For this review, take the finished solid that the model builds, in its own axes (mm). A direction names the side the tool comes from. Coordinates: 2 decimals unless noted, no trailing zeros. Loops run counter-clockwise (first coordinate to the right, second up) from the corner with the lowest first, then second, coordinate; pieces in that order, holes last. Notation, with made-up numbers: M -21.75,-28.5 L 17.25,-28.5 A21 cw 17.25,-12.5 Z; hole C -26,-34.75 d4. An arc over 180 degrees is marked long. Answer as a JSON object with one key per item and string values. Group by question number.
Item 1: Tool access review of faces 4 (the face through (6.35, 121, 10)), 5 (the face through (3, 86.995, 13)), 6 (the face through (24.99, 5.63, -55.48)): name each direction out of +Z, -Z, +X, -X, +Y, -Y from which nothing blocks a thin tool from reaching the whole face with its end or side.
Item 2: Wall thickness on L1, parallel to X at y = 66.5, z = -83; L2, parallel to Z at x = 23, y = 29.5: over which ranges is each line inside the solid? List them lowest first. Write a range as from..to.
Item 3: Add section D-D (y = 56.5). State the section outline as (x, z) points, then the cut area to 3 significant figures.
Item 4: Add section B-B (z = 4.5). State the section outline as (x, y) points (3 decimals), then the cut area to 3 significant figures.
Item 5: Insertion check: pin 1 (5 mm diameter, centred on y = 148.91, z = -92.52, fed in from -X); pin 2 (5 mm diameter, centred on x = 20, z = 14.732, fed in from +Y); pin 3 (1.9 mm diameter, centred on x = 1.5, z = 10.5, fed in from -Y) (3 decimals); pin 4 (1.5 mm diameter, centred on x = 24, z = -52.5, fed in from -Y). Each pin has a flat end and moves straight along its axis. Give the tip position at first contact, or say it passes through.
Item 6: Add section C-C (x = 24). State the section outline as (y, z) points (3 decimals), then the cut area to 3 significant figures.
Item 7: Add section A-A (x = 11). State the section outline as (y, z) points, then the cut area to 3 significant figures.
Item 8: Mouldability with a two-part tool opening along Z and no side actions: class faces 1 (the face through (8, 6, -74)), 2 (the face through (3, 65, 19.05)), 3 (the face through (3, 114.935, 13)) as +Z half, -Z half, draft (parallel to the pull), parting line (faces both ways), or undercut.
from build123d import *

# Parameters (mm, degrees)
SKETCH1_R                       = 2.54
BOSS_EXTRUDE1_DEPTH             = 11.43
BOSS_EXTRUDE2_DEPTH             = 107.95
SKETCH3_W                       = 38.1
SKETCH3_H                       = 91.186
BOSS_EXTRUDE3_DEPTH             = 35.56
CUT_EXTRUDE1_REACH              = 93.186
SKETCH4_R                       = 5.715
SKETCH5_W                       = 6.35
SKETCH5_H                       = 12.065
BOSS_EXTRUDE4_DEPTH             = 12.7
F_1_4_0_25_DIAMETER_HOLE2_D     = 6.35
F_1_4_0_25_DIAMETER_HOLE2_DEPTH = 6.351
LPATTERN2_COUNT                 = 5
LPATTERN2_PITCH                 = 27.94
SKETCH13_W                      = 6.35
SKETCH13_H                      = 11.43
BOSS_EXTRUDE5_DEPTH             = 12.7
F_1_4_0_25_DIAMETER_HOLE3_D     = 6.35
F_1_4_0_25_DIAMETER_HOLE3_DEPTH = 6.35
SKETCH16_W                      = 6.35
SKETCH16_H                      = 12.065
BOSS_EXTRUDE6_DEPTH             = 12.7
F_1_4_0_25_DIAMETER_HOLE4_D     = 6.35
F_1_4_0_25_DIAMETER_HOLE4_DEPTH = 6.35
SKETCH19_W                      = 6.35
SKETCH19_H                      = 12.065
BOSS_EXTRUDE7_DEPTH             = 12.7
F_1_4_0_25_DIAMETER_HOLE5_D     = 6.35
F_1_4_0_25_DIAMETER_HOLE5_DEPTH = 6.35
CHAMFER1_SIZE                   = 25.4
TAP_DRILL_FOR_M5X0_8_TAP1_D     = 4.2
TAP_DRILL_FOR_M5X0_8_TAP1_DEPTH = 11.43
CUT_EXTRUDE2_REACH              = 156.94
SKETCH24_R                      = 8


with BuildPart() as part:
    # Sketch1 → Boss-Extrude1 (new body)
    with BuildSketch(Plane(origin=(0, 0, 0), x_dir=(1, 0, 0), z_dir=(0, 1, 0))):
        with BuildLine():
            Line((0, 0), (14.605, 0))
            ThreePointArc((14.605, 0), (21.080049256, 8.637950744), (29.718, 15.113))
            Line((29.718, 15.113), (29.718, 44.323))
            ThreePointArc((29.718, 44.323), (21.080049256, 50.798049256), (14.605, 59.436))
            Line((14.605, 59.436), (0, 59.436))
            Line((0, 59.436), (0, 84.836))
            Line((0, 84.836), (38.1, 84.836))
            Line((38.1, 84.836), (38.1, -25.4))
            Line((38.1, -25.4), (0, -25.4))
            Line((0, -25.4), (0, 0))
        make_face()
        with Locations((23.622, 6.096)):
            Circle(SKETCH1_R, mode=Mode.SUBTRACT)
        with Locations((23.622, 53.34)):
            Circle(SKETCH1_R, mode=Mode.SUBTRACT)
    extrude(amount=BOSS_EXTRUDE1_DEPTH)

    # Sketch2 → Boss-Extrude2 (add)
    with BuildSketch(Plane(origin=(0, 11.43, 0), x_dir=(1, 0, 0), z_dir=(0, 1, 0))):
        Polygon((38.1, 84.836), (29.718, 84.836), (29.718, 0), (0, 0), (0, -6.35), (38.1, -6.35), align=None)
    extrude(amount=BOSS_EXTRUDE2_DEPTH)

    # Sketch3 → Boss-Extrude3 (add)
    with BuildSketch(Plane(origin=(0, 119.38, 0), x_dir=(1, 0, 0), z_dir=(0, 1, 0))):
        with Locations((19.05, 39.243)):
            Rectangle(SKETCH3_W, SKETCH3_H)
    extrude(amount=BOSS_EXTRUDE3_DEPTH)

    # Sketch4 → Cut-Extrude1 (cut, up to next)
    with BuildSketch(Plane.XY.offset(6.35), mode=Mode.PRIVATE) as cut_extrude1_sk1:
        with Locations((0, 137.16)):
            Circle(SKETCH4_R)
    cut_extrude1_tool1 = extrude(cut_extrude1_sk1.sketch, amount=-CUT_EXTRUDE1_REACH, mode=Mode.PRIVATE) & part.part
    add(cut_extrude1_tool1.solids().sort_by_distance((0, 137.16, 6.35))[0], mode=Mode.SUBTRACT)

    # Sketch5 → Boss-Extrude4 (add)
    with BuildSketch(Plane.XY.offset(6.35)):
        with Locations((3.175, 148.9075)):
            Rectangle(SKETCH5_W, SKETCH5_H)
    boss_extrude4 = extrude(amount=BOSS_EXTRUDE4_DEPTH)

    # 1/4 (0.25) Diameter Hole2
    with Locations(Plane(origin=(6.35, 0, 0), x_dir=(0, 0, -1), z_dir=(1, 0, 0))):
        with Locations((-13.97, 149.225)):
            f_1_4_0_25_diameter_hole2 = Hole(F_1_4_0_25_DIAMETER_HOLE2_D / 2, depth=F_1_4_0_25_DIAMETER_HOLE2_DEPTH)

    # LPattern2: Boss-Extrude4, 1/4 (0.25) Diameter Hole2 ×5
    with Locations(*[(0, -i * LPATTERN2_PITCH, 0) for i in range(1, LPATTERN2_COUNT)]):
        add(boss_extrude4)
        add(f_1_4_0_25_diameter_hole2, mode=Mode.SUBTRACT)

    # Sketch13 → Boss-Extrude5 (add)
    with BuildSketch(Plane(origin=(0, 0, -84.836), x_dir=(-1, 0, 0), z_dir=(0, 0, -1))):
        with Locations((-3.175, 5.715)):
            Rectangle(SKETCH13_W, SKETCH13_H)
    extrude(amount=BOSS_EXTRUDE5_DEPTH)

    # 1/4 (0.25) Diameter Hole3
    with Locations(Plane(origin=(6.35, 0, 0), x_dir=(0, 0, -1), z_dir=(1, 0, 0))):
        with Locations((92.456, 5.715)):
            Hole(F_1_4_0_25_DIAMETER_HOLE3_D / 2, depth=F_1_4_0_25_DIAMETER_HOLE3_DEPTH)

    # Sketch16 → Boss-Extrude6 (add)
    with BuildSketch(Plane(origin=(0, 0, -84.836), x_dir=(-1, 0, 0), z_dir=(0, 0, -1))):
        with Locations((-3.175, 148.9075)):
            Rectangle(SKETCH16_W, SKETCH16_H)
    extrude(amount=BOSS_EXTRUDE6_DEPTH)

    # 1/4 (0.25) Diameter Hole4
    with Locations(Plane(origin=(6.35, 0, 0), x_dir=(0, 0, -1), z_dir=(1, 0, 0))):
        with Locations((92.515604356, 148.9075)):
            Hole(F_1_4_0_25_DIAMETER_HOLE4_D / 2, depth=F_1_4_0_25_DIAMETER_HOLE4_DEPTH)

    # Sketch19 → Boss-Extrude7 (add)
    with BuildSketch(Plane(origin=(0, 0, -84.836), x_dir=(-1, 0, 0), z_dir=(0, 0, -1))):
        with Locations((-3.175, 125.4125)):
            Rectangle(SKETCH19_W, SKETCH19_H)
    extrude(amount=BOSS_EXTRUDE7_DEPTH)

    # 1/4 (0.25) Diameter Hole5
    with Locations(Plane(origin=(6.35, 0, 0), x_dir=(0, 0, -1), z_dir=(1, 0, 0))):
        with Locations((92.456, 125.4125)):
            Hole(F_1_4_0_25_DIAMETER_HOLE5_D / 2, depth=F_1_4_0_25_DIAMETER_HOLE5_DEPTH)

    # Chamfer1
    chamfer1_edges = [part.edges().sort_by_distance(p)[0] for p in [
        (38.1, 154.94, -39.243),
    ]]
    chamfer(chamfer1_edges, length=CHAMFER1_SIZE)

    # Tap Drill for M5x0.8 Tap1
    with Locations(Plane(origin=(0, 0, 0), x_dir=(-1, 0, 0), z_dir=(0, -1, 0))):
        with Locations((-20, 74.168), (-20, -14.732)):
            Hole(TAP_DRILL_FOR_M5X0_8_TAP1_D / 2, depth=TAP_DRILL_FOR_M5X0_8_TAP1_DEPTH)

    # Sketch24 → Cut-Extrude2 (cut, up to next)
    with BuildSketch(Plane.XZ, mode=Mode.PRIVATE) as cut_extrude2_sk1:
        with Locations((0, -74.168)):
            Circle(SKETCH24_R)
    cut_extrude2_tool1 = extrude(cut_extrude2_sk1.sketch, amount=-CUT_EXTRUDE2_REACH, mode=Mode.PRIVATE) & part.part
    add(cut_extrude2_tool1.solids().sort_by_distance((0, 0, -74.168))[0], mode=Mode.SUBTRACT)
    # Sketch24 → Cut-Extrude2 (cut, up to next)
    with BuildSketch(Plane.XZ, mode=Mode.PRIVATE) as cut_extrude2_sk2:
        with Locations((0, 14.732)):
            Circle(SKETCH24_R)
    cut_extrude2_tool2 = extrude(cut_extrude2_sk2.sketch, amount=-CUT_EXTRUDE2_REACH, mode=Mode.PRIVATE) & part.part
    add(cut_extrude2_tool2.solids().sort_by_distance((0, 0, 14.732))[0], mode=Mode.SUBTRACT)


solid = part.part
From the geometry:
{
 "1": {"face 4": "+Z, +X, +Y", "face 5": "+Z, +X, -X", "face 6": "-Y"},
 "2": {"L1": "x = 29.72..38.1", "L2": "z = 0..6.35"},
 "3": {"outline": "M 0,0 L 29.72,0 L 29.72,-84.84 L 38.1,-84.84 L 38.1,6.35 L 0,6.35 Z", "area": "953 mm²"},
 "4": {"outline": "M 0,0 L 38.1,0 L 38.1,129.54 L 12.7,154.94 L 0,154.94 L 0,142.875 A5.715 cw 0,131.445 Z", "area": "5,530 mm²"},
 "5": {"pin 1": "passes through", "pin 2": "stops at y = 11.43", "pin 3": "stops at y = 31.115", "pin 4": "stops at y = 119.38"},
 "6": {"outline": "M 0,-84.836 L 11.43,-84.836 L 11.43,-55.852 L 0,-55.852 Z; M 0,-50.828 L 11.43,-50.828 L 11.43,-48.165 L 0,-48.165 Z; M 0,-11.271 L 11.43,-11.271 L 11.43,-8.608 L 0,-8.608 Z; M 0,-3.584 L 11.43,-3.584 L 11.43,0 L 119.38,0 L 119.38,-84.836 L 143.64,-84.836 L 143.64,6.35 L 11.43,6.35 L 11.43,25.4 L 0,25.4 Z", "area": "3,620 mm²"},
 "7": {"outline": "M 0,-84.84 L 11.43,-84.84 L 11.43,-59.44 L 0,-59.44 Z; M 0,0 L 119.38,0 L 119.38,-84.84 L 154.94,-84.84 L 154.94,6.35 L 11.43,6.35 L 11.43,25.4 L 0,25.4 Z", "area": "4,510 mm²"},
 "8": {"face 1": "undercut", "face 2": "+Z half", "face 3": "draft"}
}
